Verification items for this drawing (mm, ordinates from the low corner). A direction names the side the tool comes from. Round coordinates to 2 decimals unless told otherwise and drop trailing zeros. Order: outer loops, then holes, each group sorted by start corner. A loop starts at its lowest first (then second) coordinate and runs counter-clockwise, first axis right, second up. Notation, with made-up numbers: (57, -40) -> (67, -40) arc R22 ccw to (67, -13) -> close; hole circle Ø1 at (-1.75, 30.5). An arc over 180 degrees is marked (long way). Answer in a Markdown table with one row per item.
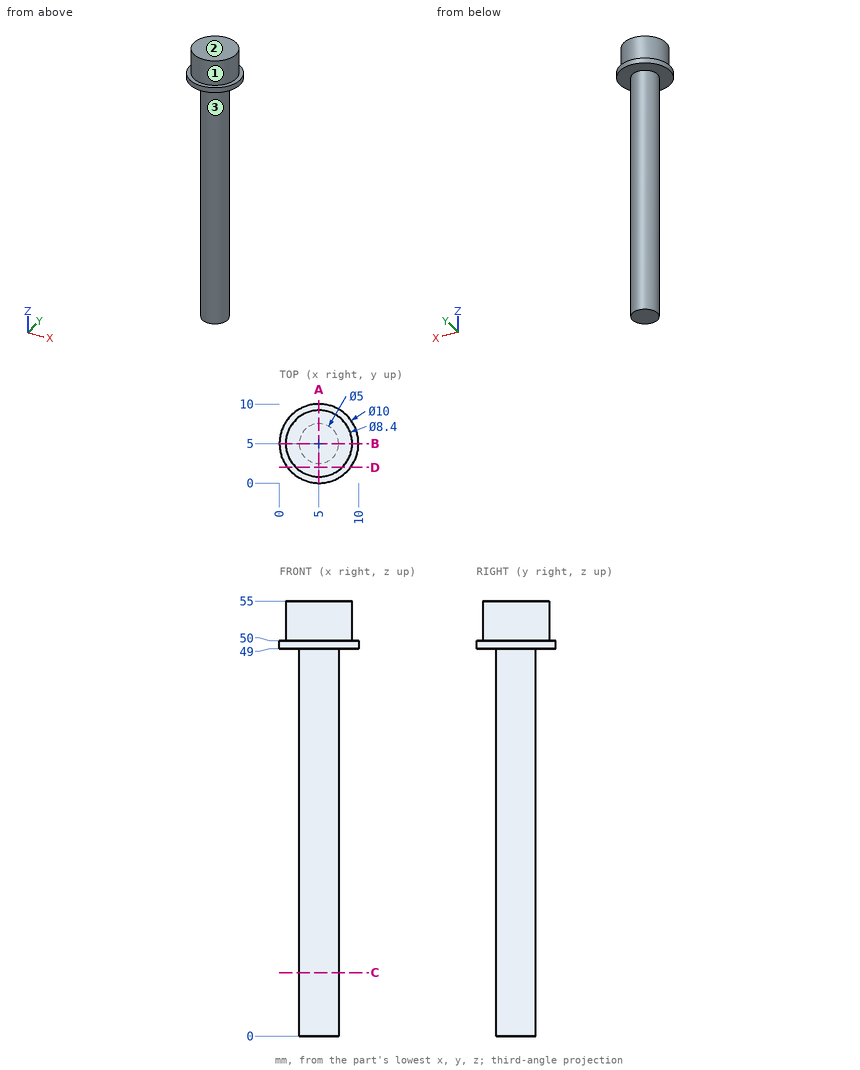
Item 1: Set-up check for the marked faces 1, 2 and 3: record each of +Z, -Z, +X, -X, +Y, -Y from which the full face is reachable in a straight line by a thin tool's end or side.
Result sheet:
| item | result |
|---|---|
| face 1 | +Z |
| face 2 | +Z, +X, -X, +Y, -Y |
| face 3 | -Z |
Item 2: Cross-section at C-C (z = 8). Record the boundary of the cut face in (x, y).
Result sheet:
| item | result |
|---|---|
| outline | circle Ø5 at (5, 5) |
Item 3: Depth check by flat-ended pin: P1, Ø2, axis at x = 6.5, z = 40, coming from the +Y side; P2, Ø6, axis at x = 2, z = 21, coming from the -Y side; P3, Ø5, axis at y = 8, z = 15, coming from the +X side. Enter the tip coordinate at first touch or a pass-through.
Result sheet:
| item | result |
|---|---|
| P1 | stops at y = 7.45 |
| P2 | stops at y = 2.5 |
| P3 | stops at x = 7.45 |
Item 4: Cross-section at A-A (x = 5). Record the boundary of the cut face in (y, z), and give its area (3 significant figures).
Result sheet:
| item | result |
|---|---|
| outline | (0, 49) -> (2.5, 49) -> (2.5, 0) -> (7.5, 0) -> (7.5, 49) -> (10, 49) -> (10, 50) -> (9.2, 50) -> (9.2, 55) -> (0.8, 55) -> (0.8, 50) -> (0, 50) -> close |
| area | 297 mm^2 |
Item 5: Scan lines: line 1 (Z direction, x = 4.75, y = 1.5); line 2 (Y direction, x = 5, z = 6); line 3 (Z direction, x = 5.25, y = 0.5). Record each from-to range of solid material in increasing order. Write a range as [from, to].
Result sheet:
| item | result |
|---|---|
| line 1 | z = [49, 55] |
| line 2 | y = [2.5, 7.5] |
| line 3 | z = [49, 50] |
Item 6: Cross-section at D-D (y = 2). Record the boundary of the cut face in (x, z).
Result sheet:
| item | result |
|---|---|
| outline | (1, 49) -> (9, 49) -> (9, 50) -> (7.94, 50) -> (7.94, 55) -> (2.06, 55) -> (2.06, 50) -> (1, 50) -> close |
